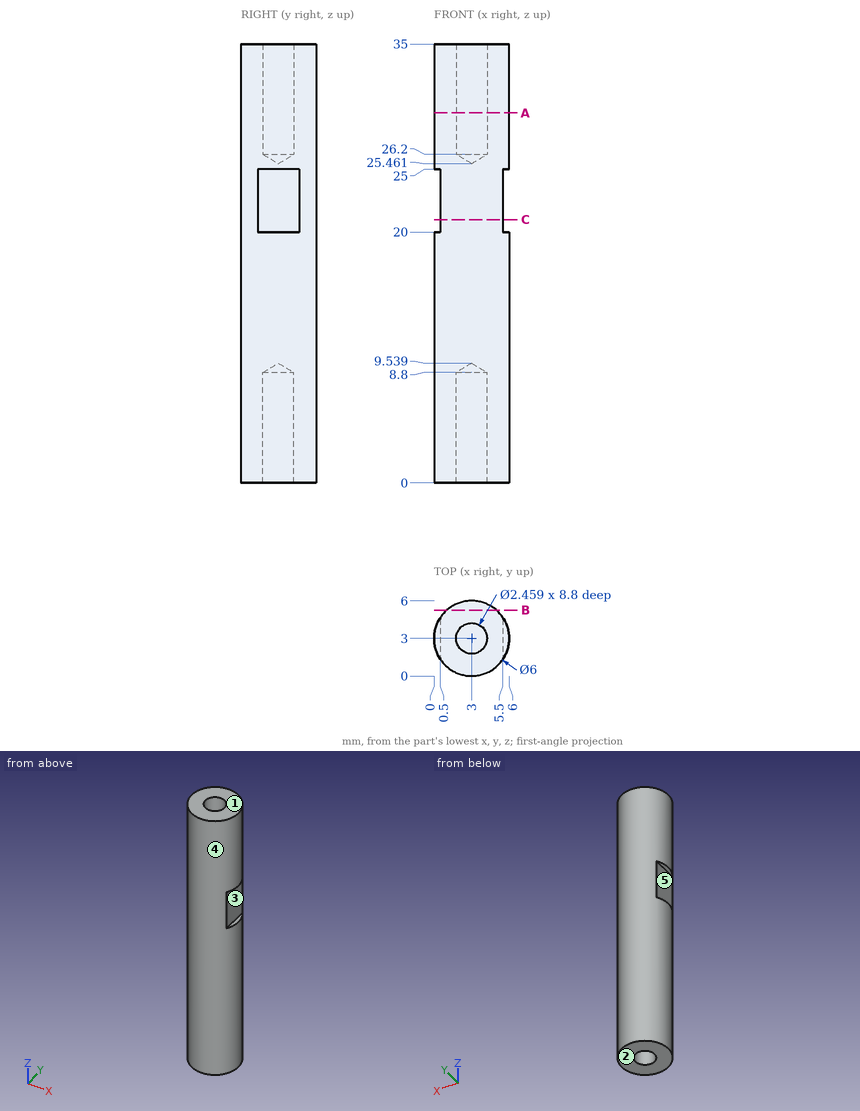
Input: dimensioned drawing with shaded views. Units: mm. Origin: part minimum x, y, z. A direction names the side the tool comes from. Give positions to 0.01 mm unless a question says otherwise; leave off trailing zeros. Write each loop counter-clockwise with the first axis right and the second up, starting at its lowest first coordinate (ties: lowest second). Pieces come first, ordered by that corner, then holes.
1. Material intervals for line 1 along X through (y, z) = (3, 33.25); line 2 along Z through (x, y) = (5.6, 1.8); line 3 along Y through (x, z) = (2.05, 32.5) (1 decimal), sorted ascending.
2. First-contact query: pin 1 (2 mm diameter, centred on y = 1, z = 23.5, fed in from -X); pin 2 (3 mm diameter, centred on y = 5, z = 11, fed in from -X); pin 3 (1 mm diameter, centred on y = 1, z = 13.5, fed in from +X). Flat tips, straight axial feed; report the tip coordinate or a pass-through.
3. Section query C-C (z = 21). Return the cut outline in (x, y).
4. Pull-direction query (Z, two-part tool) for the marked faces 1, 2 and 3; classes: +Z half, -Z half, draft (parallel to the pull), parting line (faces both ways), or undercut.
5. Access query for the marked faces 4 and 5. Directions: +Z, -Z, +X, -X, +Y, -Y. A direction counts if a zero-diameter tool reaches every point of the face in a straight line with its end or side. Return the directions, or none.
6. Section query B-B (y = 5.25). Return the cut outline in (x, z), then the cut area to 3 significant figures.
7. Section query A-A (z = 29.5). Return the cut outline in (x, y).
Output values:
1. line 1: x = 0 to 1.77, 4.23 to 6
1. line 2: z = 0 to 20, 25 to 35
1. line 3: y = 0.2 to 2.2, 3.8 to 5.8
2. pin 1: stops at x = 0.5
2. pin 2: stops at x = 0.04
2. pin 3: stops at x = 5.6
3. outline: (0.5, 1.34) arc R3 ccw to (5.5, 1.34) - (5.5, 4.66) arc R3 ccw to (0.5, 4.66) - close
4. face 1: +Z half
4. face 2: -Z half
4. face 3: undercut
5. face 4: +Z, -Z
5. face 5: -X, +Y, -Y
6. outline: (1.02, 0) - (4.98, 0) - (4.98, 35) - (1.02, 35) - close
6. area: 139 mm2
7. outline: circle Ø6 at (3, 3); hole circle Ø2.46 at (3, 3)
